```python
from build123d import *

# Parameters (mm, degrees)
F0_W     = 17.78
F0_H     = 17.78
F0_R     = 8.001
F1_DEPTH = 3.81


with BuildPart() as f1:
    # F0 (on Top) → F1 (new body)
    with BuildSketch(Plane.XY):
        Polygon((-8.89, 8.89), (8.89, 8.89), (0, 32.683442), align=None)
        Polygon((-8.89, -8.89), (-8.89, 8.89), (-32.683442, 0), align=None)
        Polygon((0, -32.683442), (8.89, -8.89), (-8.89, -8.89), align=None)
        Polygon((32.683442, 0), (8.89, 8.89), (8.89, -8.89), align=None)
        Rectangle(F0_W, F0_H)
        Circle(F0_R, mode=Mode.SUBTRACT)
    extrude(amount=F1_DEPTH)


solid = f1.part
```
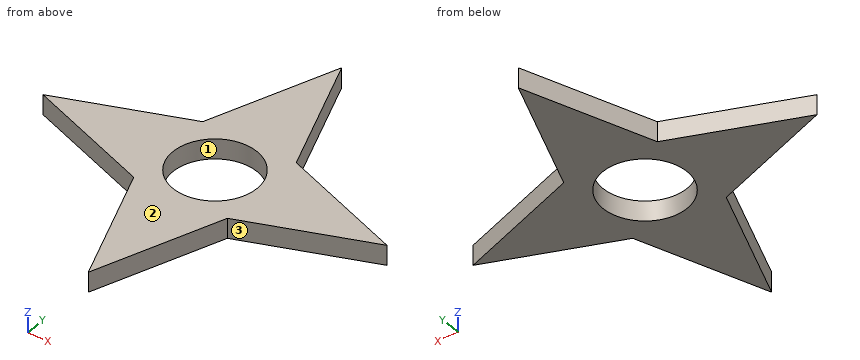
The listing builds one solid part. Answer for the finished solid, in the listing's coordinates (mm). Face numbers are marked on the shaded views. Round coordinates to 2 decimals unless told otherwise and drop trailing zeros. Loops run counter-clockwise (first coordinate to the right, second up) from the corner with the lowest first, then second, coordinate; pieces in that order, holes last. Notation, with made-up numbers: (52, 57) - (64, 57) arc R32 ccw to (64, 87) - close; hole circle Ø1 at (-38, 79.5). An arc over 180 degrees is marked (long way). Use one line per item in the form item = value. Start each with the question number.
1. The part is cut by section A-A on z = 1.25. Determine the outline of the cut face in (x, y).
2. For a pull along Y with two mould halves and no side action, classify the marked faces 1, 2 and 3 as pulls with the +Y half, pulls with the -Y half, needs draft (parallel to the pull), parting line crosses it, or undercut.
3. The part is cut by section D-D on y = -13. Determine the outline of the cut face in (x, z), then the cut area to 3 significant figures.
4. Given pin 1 Ø13 at (x, y) = (0, 0) entering from -Z; pin 2 Ø1.5 at (y, z) = (12, 2) entering from -X, each flat-ended and moving along its own axis, determine where each tip first touches the part or whether it passes through.
5. Consider line 1 (X direction, y = 21, z = 1.3); line 2 (Y direction, x = -15, z = 2); line 3 (X direction, y = -23, z = 3.05). Determine where each line is inside the solid, lowest interval first. Write a range as [from, to].
6. The part is cut by section B-B on y = 4. Determine the outline of the cut face in (x, z), then the cut area to 3 significant figures.
7. The part is cut by section C-C on x = -14. Determine the outline of the cut face in (y, z).
Geometry check:
q1.outline = (-32.68, 0) - (-8.89, -8.89) - (0, -32.68) - (8.89, -8.89) - (32.68, 0) - (8.89, 8.89) - (0, 32.68) - (-8.89, 8.89) - close; hole circle Ø16 at (0, 0)
q2.face_1 = undercut
q2.face_2 = needs draft
q2.face_3 = pulls with the -Y half
q3.outline = (-7.35, 0) - (7.35, 0) - (7.35, 3.81) - (-7.35, 3.81) - close
q3.area = 56.0 mm^2
q4.pin_1 = through
q4.pin_2 = -8.01
q5.line_1 = [-4.37, 4.37]
q5.line_2 = [-6.61, 6.61]
q5.line_3 = [-3.62, 3.62]
q6.outline = (-21.98, 0) - (-6.93, 0) - (-6.93, 3.81) - (-21.98, 3.81) - close; (6.93, 0) - (21.98, 0) - (21.98, 3.81) - (6.93, 3.81) - close
q6.area = 115 mm^2
q7.outline = (-6.98, 0) - (6.98, 0) - (6.98, 3.81) - (-6.98, 3.81) - close
